Can you work these out from the model? Positions are in its coordinate system, mm. A direction names the side the tool comes from. Round coordinates to 2 decimals unless told otherwise and drop trailing zeros. Loops run counter-clockwise (first coordinate to the right, second up) from the corner with the lowest first, then second, coordinate; pieces in that order, holes last. Notation, with made-up numbers: M 46.25,4 L 76.25,4 A7 cw 76.25,14 Z; hole C 36,19 d10. An arc over 180 degrees is marked long. Return JSON: item names as keys, results as strings.
```python
from build123d import *

# Parameters (mm, degrees)
SKETCH_1_W      = 36
SKETCH_1_H      = 36
SKETCH_1_W_2    = 12
SKETCH_1_H_2    = 3.5
EXTRUDE_1_DEPTH = 5
SKETCH_2_W      = 36
SKETCH_2_H      = 36
SKETCH_2_W_2    = 28.5
SKETCH_2_H_2    = 28.5
EXTRUDE_3_DEPTH = 10
SKETCH_3_W      = 36
SKETCH_3_H      = 10
SKETCH_3_W_2    = 12
SKETCH_3_H_2    = 3.5
EXTRUDE_4_DEPTH = 16


with BuildPart() as part:
    # 草圖1 → 填料-伸長1 (new body)
    with BuildSketch(Plane(origin=(0, 0, 0), x_dir=(1, 0, 0), z_dir=(0, 1, 0))):
        Rectangle(SKETCH_1_W, SKETCH_1_H)
        with Locations((0.454747486, 12.5)):
            Rectangle(SKETCH_1_W_2, SKETCH_1_H_2, mode=Mode.SUBTRACT)
    extrude(amount=EXTRUDE_1_DEPTH)

    # 草圖2 → 填料-伸長3 (add)
    with BuildSketch(Plane(origin=(0, 0, 0), x_dir=(1, 0, 0), z_dir=(0, 1, 0))):
        Rectangle(SKETCH_2_W, SKETCH_2_H)
        Rectangle(SKETCH_2_W_2, SKETCH_2_H_2, mode=Mode.SUBTRACT)
    extrude(amount=EXTRUDE_3_DEPTH)

    # 草圖3 → 填料-伸長4 (add)
    with BuildSketch(Plane(origin=(0, 0, 0), x_dir=(1, 0, 0), z_dir=(0, 1, 0))):
        with Locations((0, 13)):
            Rectangle(SKETCH_3_W, SKETCH_3_H)
        with Locations((0.454747486, 12.5)):
            Rectangle(SKETCH_3_W_2, SKETCH_3_H_2, mode=Mode.SUBTRACT)
    extrude(amount=-EXTRUDE_4_DEPTH)


solid = part.part
```
Q1. I'm going to push flat-ended pins straight in: pin 1 Ø8 at (x, z) = (0, 8.5) entering from +Y; pin 2 Ø6 at (x, z) = (2.5, 11.5) entering from -Y; pin 3 Ø8 at (x, y) = (2, -9.5) entering from +Z. Where does each tip first touch, or does it pass through?
Results:
{"pin 1": "stops at y = 5", "pin 2": "stops at y = 0", "pin 3": "stops at z = -8"}
Q2. Suppose I cut it at B-B, the plane x = 4.5. Please give me the cut outline in (y, z).
Results:
{"outline": "M -16,-18 L 10,-18 L 10,-14.25 L -16,-14.25 Z; M -16,-10.75 L 5,-10.75 L 5,14.25 L 10,14.25 L 10,18 L 0,18 L 0,-8 L -16,-8 Z"}
Q3. Suppose I cut it at C-C, the plane x = 12. Please give me the cut outline in (y, z), plus the area to 4 significant figures.
Results:
{"outline": "M -16,-18 L 10,-18 L 10,-14.25 L 5,-14.25 L 5,14.25 L 10,14.25 L 10,18 L 0,18 L 0,-8 L -16,-8 Z", "area": "377.5 mm2"}
Q4. Suppose I cut it at A-A, the plane y = 1.25. Please give me the cut outline in (x, z).
Results:
{"outline": "M -18,-18 L 18,-18 L 18,18 L -18,18 Z; hole M -5.55,-14.25 L 6.45,-14.25 L 6.45,-10.75 L -5.55,-10.75 Z"}
Q5. On a 3-axis mill with a long thin cutter (end or side, diameter ignored), from which of +Z, -Z, +X, -X, +Y, -Y can I reach the whole of each face in a straight line? I mean faces 4 (the flat face through (18, 3, -4)), 5 (the flat face through (-5.545, -5, -12)), 6 (the flat face through (0, -8, -8)), 7 (the flat face through (-18, 3, -4)), 8 (the flat face through (-14.25, 7, 0)). Say none if no direction works.
Results:
{"face 4": "+Z, -Z, +X, +Y, -Y", "face 5": "+Y, -Y", "face 6": "+Z, +X, -X, -Y", "face 7": "+Z, -Z, -X, +Y, -Y", "face 8": "+Y"}
Q6. If I drill on line 1 along X through (y, z) = (5.5, -6.5); line 2 along X through (y, z) = (1.75, -13); line 3 along Y through (x, z) = (-6, -2.5), over which ranges is the centre line in solid material (lowest first)?
Results:
{"line 1": "x = -18 to -14.25, 14.25 to 18", "line 2": "x = -18 to -5.55, 6.45 to 18", "line 3": "y = 0 to 5"}
Q7. Thinking about a two-plate mould opening in Y: for faces 1 (the flat face through (-16, 10, 0)), 2 (the flat face through (0, -3, -18)), 3 (the flat face through (0, 0, 5)), which applies, pulls with the +Y half, pulls with the -Y half, needs draft (parallel to the pull), parting line crosses it, or undercut?
Results:
{"face 1": "pulls with the +Y half", "face 2": "needs draft", "face 3": "pulls with the -Y half"}
Q8. Suppose I cut it at D-D, the plane z = -9.5. Please give me the cut outline in (x, y), plus the area to 4 significant figures.
Results:
{"outline": "M -18,-16 L 18,-16 L 18,10 L 14.25,10 L 14.25,5 L -14.25,5 L -14.25,10 L -18,10 Z", "area": "793.5 mm2"}
